from build123d import *

# Parameters (mm, degrees)
SKETCH1_W           = 7.1
SKETCH1_H           = 6.9
BOSS_EXTRUDE1_DEPTH = 6


with BuildPart() as part:
    # Sketch1 → Boss-Extrude1 (new body)
    with BuildSketch(Plane.XY):
        Polygon((-358.994880286, -293.50655928), (-358.753699331, -293.406658857), (-358.494880286, -293.372584684), (-355.895187501, -293.372584684), (-355.636368456, -293.406658857), (-355.395187501, -293.50655928), (-355.18808072, -293.665477903), (-355.029162097, -293.872584684), (-354.929261675, -294.113765639), (-354.895187501, -294.372584684), (-354.899121361, -357.473371332), (-354.933365099, -357.732036876), (-355.033357982, -357.973038786), (-355.192292447, -358.179969532), (-355.399348154, -358.338741166), (-355.640428649, -358.438544435), (-355.899121051, -358.472584684), (-358.493457382, -358.472584684), (-358.752276427, -358.43851051), (-358.993457382, -358.338610088), (-359.200564163, -358.179691465), (-359.359482786, -357.972584684), (-359.459383208, -357.731403729), (-359.493457382, -357.472584684), (-359.493457382, -352.472584684), (-368.993457382, -352.472584684), (-368.993457382, -357.472584684), (-369.027531556, -357.731403729), (-369.127431978, -357.972584684), (-369.286350601, -358.179691465), (-369.493457382, -358.338610088), (-369.734638337, -358.43851051), (-369.993457382, -358.472584684), (-391.293457382, -358.472584684), (-391.552276427, -358.43851051), (-391.793457382, -358.338610088), (-392.000564163, -358.179691465), (-392.159482786, -357.972584684), (-392.259383208, -357.731403729), (-392.293457382, -357.472584684), (-392.293457382, -352.472584684), (-403.593457382, -352.472584684), (-403.593457382, -299.372584684), (-392.293457382, -299.372584684), (-392.293457382, -294.372584684), (-392.259383208, -294.113765639), (-392.159482786, -293.872584684), (-392.000564163, -293.665477903), (-391.793457382, -293.50655928), (-391.552276427, -293.406658857), (-391.293457382, -293.372584684), (-369.993457382, -293.372584684), (-369.734638337, -293.406658857), (-369.493457382, -293.50655928), (-369.286350601, -293.665477903), (-369.127431978, -293.872584684), (-369.027531556, -294.113765639), (-368.993457382, -294.372584684), (-368.993457382, -299.372584684), (-359.494880286, -299.372584684), (-359.494880286, -294.372584684), (-359.460806112, -294.113765639), (-359.36090569, -293.872584684), (-359.201987067, -293.665477903), align=None)
        Polygon((-357.610920971, -342.372584684), (-357.672254484, -342.838458965), (-357.852075244, -343.272584684), (-358.138128765, -343.64537689), (-358.510920971, -343.931430411), (-358.94504669, -344.111251171), (-359.410920971, -344.172584684), (-359.876795252, -344.111251171), (-360.310920971, -343.931430411), (-360.683713177, -343.64537689), (-360.969766698, -343.272584684), (-361.149587458, -342.838458965), (-361.210920971, -342.372584684), (-361.149587458, -341.906710403), (-360.969766698, -341.472584684), (-360.683713177, -341.099792478), (-360.310920971, -340.813738957), (-359.876795252, -340.633918196), (-359.410920971, -340.572584684), (-358.94504669, -340.633918196), (-358.510920971, -340.813738957), (-358.138128765, -341.099792478), (-357.852075244, -341.472584684), (-357.672254484, -341.906710403), align=None, mode=Mode.SUBTRACT)
        Polygon((-397.058387805, -347.482605219), (-396.867409445, -347.911939484), (-396.7940584, -348.376073376), (-396.843333421, -348.843376937), (-397.011876498, -349.282004201), (-397.288201699, -349.662063445), (-397.653477917, -349.95765426), (-398.082812183, -350.148632621), (-398.546946075, -350.221983666), (-399.014249636, -350.172708645), (-399.4528769, -350.004165568), (-399.832936144, -349.727840367), (-400.128526959, -349.362564149), (-400.319505319, -348.933229883), (-400.392856365, -348.469095991), (-400.343581343, -348.00179243), (-400.175038266, -347.563165166), (-399.898713066, -347.183105922), (-399.533436847, -346.887515107), (-399.104102582, -346.696536747), (-398.63996869, -346.623185701), (-398.172665129, -346.672460723), (-397.734037865, -346.8410038), (-397.35397862, -347.117329), align=None, mode=Mode.SUBTRACT)
        with Locations((-395.260918473, -310.622584684)):
            Rectangle(SKETCH1_W, SKETCH1_H, mode=Mode.SUBTRACT)
        Polygon((-375.710923469, -337.772584684), (-368.342459311, -337.772584684), (-368.342459311, -344.672584684), (-375.710923469, -344.672584684), (-375.710923469, -350.922574533), (-386.710918473, -350.922574533), (-386.710918473, -300.922594835), (-375.710923469, -300.922594835), (-375.710923469, -307.172584684), (-368.342459311, -307.172584684), (-368.342459311, -314.072584684), (-375.710923469, -314.072584684), align=None, mode=Mode.SUBTRACT)
        Polygon((-358.138128765, -310.74537689), (-358.510920971, -311.031430411), (-358.94504669, -311.211251171), (-359.410920971, -311.272584684), (-359.876795252, -311.211251171), (-360.310920971, -311.031430411), (-360.683713177, -310.74537689), (-360.969766698, -310.372584684), (-361.149587458, -309.938458965), (-361.210920971, -309.472584684), (-361.149587458, -309.006710403), (-360.969766698, -308.572584684), (-360.683713177, -308.199792478), (-360.310920971, -307.913738957), (-359.876795252, -307.733918196), (-359.410920971, -307.672584684), (-358.94504669, -307.733918196), (-358.510920971, -307.913738957), (-358.138128765, -308.199792478), (-357.852075244, -308.572584684), (-357.672254484, -309.006710403), (-357.610920971, -309.472584684), (-357.672254484, -309.938458965), (-357.852075244, -310.372584684), align=None, mode=Mode.SUBTRACT)
        Polygon((-400.321176702, -303.927546021), (-400.392999705, -303.463173217), (-400.342186872, -302.99603437), (-400.172201015, -302.557964223), (-399.894626388, -302.178816531), (-399.528379244, -301.884429584), (-399.09841872, -301.694865364), (-398.634045915, -301.623042361), (-398.166907069, -301.673855193), (-397.728836921, -301.843841051), (-397.34968923, -302.121415678), (-397.055302282, -302.487662822), (-396.865738063, -302.917623346), (-396.79391506, -303.381996151), (-396.844727892, -303.849134997), (-397.014713749, -304.287205145), (-397.292288376, -304.666352836), (-397.65853552, -304.960739784), (-398.088496044, -305.150304003), (-398.552868849, -305.222127006), (-399.020007696, -305.171314174), (-399.458077843, -305.001328317), (-399.837225535, -304.72375369), (-400.131612482, -304.357506546), align=None, mode=Mode.SUBTRACT)
        with Locations((-395.260918473, -341.222584684)):
            Rectangle(SKETCH1_W, SKETCH1_H, mode=Mode.SUBTRACT)
    extrude(amount=BOSS_EXTRUDE1_DEPTH)


solid = part.part
Can you work these out from the model? Positions are in its coordinate system, mm. A direction names the side the tool comes from. Round coordinates to 2 decimals unless told otherwise and drop trailing zeros. Order: outer loops, then holes, each group sorted by start corner. A loop starts at its lowest first (then second) coordinate and runs counter-clockwise, first axis right, second up. Notation, with made-up numbers: M -32.5,-20 L 4.5,-20 A26 ccw 4.5,19 Z; hole C -4.75,13 d11. An arc over 180 degrees is marked long. Use a Markdown table: item, result.
1) If we mould it in two halves opening along X, with no side actions, what happens to faces 4 (the face through (-395, -337.773, 3)), 5 (the face through (-373, -325, 0))? For each: +X half, -X half, draft (parallel to the pull), parting line (faces both ways), or undercut.
Geometry says:
| item | result |
|---|---|
| face 4 | undercut |
| face 5 | draft |
2) Imagine slicing it at B-B (x = -383). List the corners of the cut face in (y, z) for me, then the cut area to 3 significant figures.
Geometry says:
| item | result |
|---|---|
| outline | M -358.47,0 L -350.92,0 L -350.92,6 L -358.47,6 Z; M -300.92,0 L -293.37,0 L -293.37,6 L -300.92,6 Z |
| area | 90.6 mm² |
3) Imagine slicing it at C-C (y = -315). List the corners of the cut face in (x, z) for me.
Geometry says:
| item | result |
|---|---|
| outline | M -403.59,0 L -386.71,0 L -386.71,6 L -403.59,6 Z; M -375.71,0 L -354.9,0 L -354.9,6 L -375.71,6 Z |
4) I'm going to push flat-ended pins straight in: P1, Ø3, axis at x = -399.5, z = 3.5, coming from the +Y side; P2, Ø1, axis at x = -397.5, z = 2, coming from the -Y side; P3, Ø2.5, axis at y = -296.5, z = 2.5, coming from the -X side; P4, Ø6, axis at x = -383, y = -302.5, coming from the +Z side. Where does each tip first touch, or does it pass through?
Geometry says:
| item | result |
|---|---|
| P1 | stops at y = -299.37 |
| P2 | stops at y = -352.47 |
| P3 | stops at x = -392.29 |
| P4 | stops at z = 6 |
5) Imagine slicing it at A-A (x = -393). List the corners of the cut face in (y, z) for me.
Geometry says:
| item | result |
|---|---|
| outline | M -352.47,0 L -344.67,0 L -344.67,6 L -352.47,6 Z; M -337.77,0 L -314.07,0 L -314.07,6 L -337.77,6 Z; M -307.17,0 L -299.37,0 L -299.37,6 L -307.17,6 Z |
6) If I drill on line 1 along Y through (x, z) = (-371, 5); line 2 along X through (y, z) = (-314, 5.15); line 3 along Y through (x, z) = (-369.5, 3.05), over which ranges is the centre line in solid material (lowest first)?
Geometry says:
| item | result |
|---|---|
| line 1 | y = -358.47 to -344.67, -337.77 to -314.07, -307.17 to -293.37 |
| line 2 | x = -403.59 to -398.81, -391.71 to -386.71, -368.34 to -354.9 |
| line 3 | y = -358.34 to -344.67, -337.77 to -314.07, -307.17 to -293.5 |
7) On a 3-axis mill with a long thin cutter (end or side, diameter ignored), from which of +Z, -Z, +X, -X, +Y, -Y can I reach the whole of each face in a straight line? I mean faces 1 (the face through (-359.493, -355, 3)), 2 (the face through (-398.811, -341, 3)), 3 (the face through (-398, -352.473, 3)). Say none if no direction works.
Geometry says:
| item | result |
|---|---|
| face 1 | +Z, -Z, -Y |
| face 2 | +Z, -Z |
| face 3 | +Z, -Z, -X, -Y |
8) Imagine slicing it at D-D (z = 2.15). Give the number of separate pieces and of enclosed holes in the cut face, then the cut area to 3 significant figures.
Geometry says:
| item | result |
|---|---|
| separate pieces | 1 |
| enclosed holes | 7 |
| area | 2,130 mm² |
